```python
from build123d import *

# Parameters (mm, degrees)
SKETCH1_R           = 50.8
BOSS_EXTRUDE1_DEPTH = 15.875
CUT_EXTRUDE2_DEPTH  = 15.24
SKETCH5_R           = 4.191
CUT_EXTRUDE3_DEPTH  = 74.440708058
CUT_EXTRUDE4_DEPTH  = 74.575101937
SKETCH7_R           = 48.26
CUT_EXTRUDE5_DEPTH  = 15.24
SKETCH8_R           = 3.2639
CUT_EXTRUDE6_DEPTH  = 74.575101937


with BuildPart() as part:
    # Sketch1 → Boss-Extrude1 (new body)
    with BuildSketch(Plane(origin=(0, 0, 0), x_dir=(1, 0, 0), z_dir=(0, 1, 0))):
        with Locations(Location((0, 0, 0), (0, 0, 270))):
            Circle(SKETCH1_R)
    extrude(amount=BOSS_EXTRUDE1_DEPTH)

    # Sketch4 → Cut-Extrude2 (cut)
    with BuildSketch(Plane(origin=(0, 15.875, 0), x_dir=(1, 0, 0), z_dir=(0, 1, 0))):
        Polygon((-3.519527241, 6.096), (3.519527241, 6.096), (7.039054482, 0), (3.519527241, -6.096), (-3.519527241, -6.096), (-7.039054482, 0), align=None)
    extrude(amount=-CUT_EXTRUDE2_DEPTH, mode=Mode.SUBTRACT)

    # Sketch5 → Cut-Extrude3 (cut, through all)
    with BuildSketch(Plane(origin=(0, 0.635, 0), x_dir=(1, 0, 0), z_dir=(0, 1, 0))):
        with Locations(Location((0, 0, 0), (0, 0, 270))):
            Circle(SKETCH5_R)
    extrude(amount=-CUT_EXTRUDE3_DEPTH, mode=Mode.SUBTRACT)

    # Sketch6 → Cut-Extrude4 (cut, through all)
    with BuildSketch(Plane(origin=(0, 15.875, 0), x_dir=(1, 0, 0), z_dir=(0, 1, 0))):
        with BuildLine():
            ThreePointArc((-13.470384182, 13.470384182), (-7.290119387, 17.599905094), (0, 19.05))
            Line((0, 19.05), (0, 38.1))
            ThreePointArc((0, 38.1), (-14.580238773, 35.199810189), (-26.940768363, 26.940768363))
            Line((-26.940768363, 26.940768363), (-13.470384182, 13.470384182))
        make_face()
        with BuildLine():
            Line((26.940768363, 26.940768363), (13.470384182, 13.470384182))
            ThreePointArc((13.470384182, 13.470384182), (17.599905094, 7.290119387), (19.05, 0))
            Line((19.05, 0), (38.1, 0))
            ThreePointArc((38.1, 0), (35.199810189, 14.580238773), (26.940768363, 26.940768363))
        make_face()
        with BuildLine():
            Line((26.940768363, -26.940768363), (13.470384182, -13.470384182))
            ThreePointArc((13.470384182, -13.470384182), (7.290119387, -17.599905094), (0, -19.05))
            Line((0, -19.05), (0, -38.1))
            ThreePointArc((0, -38.1), (14.580238773, -35.199810189), (26.940768363, -26.940768363))
        make_face()
        with BuildLine():
            Line((-26.940768363, -26.940768363), (-13.470384182, -13.470384182))
            ThreePointArc((-13.470384182, -13.470384182), (-17.599905094, -7.290119387), (-19.05, 0))
            Line((-19.05, 0), (-38.1, 0))
            ThreePointArc((-38.1, 0), (-35.199810189, -14.580238773), (-26.940768363, -26.940768363))
        make_face()
    extrude(amount=-CUT_EXTRUDE4_DEPTH, mode=Mode.SUBTRACT)

    # Sketch7 → Cut-Extrude5 (cut)
    with BuildSketch(Plane(origin=(0, 15.875, 0), x_dir=(1, 0, 0), z_dir=(0, 1, 0))):
        with Locations(Location((0, 0, 0), (0, 0, 270))):
            Circle(SKETCH7_R)
        with BuildLine():
            Line((-16.313445375, 2.54), (-40.560547334, 2.54))
            ThreePointArc((-40.560547334, 2.54), (-37.546464201, -15.552254691), (-26.884586844, -30.476689292))
            Line((-26.884586844, -30.476689292), (-9.739296625, -13.331399073))
            ThreePointArc((-9.739296625, -13.331399073), (-15.253251082, -6.318103468), (-16.313445375, 2.54))
        make_face(mode=Mode.SUBTRACT)
        with BuildLine():
            Line((16.313445375, -2.54), (40.560547334, -2.54))
            ThreePointArc((40.560547334, -2.54), (37.546464201, 15.552254691), (26.884586844, 30.476689292))
            Line((26.884586844, 30.476689292), (9.739296625, 13.331399073))
            ThreePointArc((9.739296625, 13.331399073), (15.253251082, 6.318103468), (16.313445375, -2.54))
        make_face(mode=Mode.SUBTRACT)
        Polygon((4.985996925, 8.636), (-4.985996925, 8.636), (-9.971993849, 0), (-4.985996925, -8.636), (4.985996925, -8.636), (9.971993849, 0), align=None, mode=Mode.SUBTRACT)
        with BuildLine():
            ThreePointArc((2.54, 40.560547334), (-15.552254691, 37.546464201), (-30.476689292, 26.884586844))
            Line((-30.476689292, 26.884586844), (-13.331399073, 9.739296625))
            ThreePointArc((-13.331399073, 9.739296625), (-6.318103468, 15.253251082), (2.54, 16.313445375))
            Line((2.54, 16.313445375), (2.54, 40.560547334))
        make_face(mode=Mode.SUBTRACT)
        with BuildLine():
            Line((-2.54, -16.313445375), (-2.54, -40.560547334))
            ThreePointArc((-2.54, -40.560547334), (15.552254691, -37.546464201), (30.476689292, -26.884586844))
            Line((30.476689292, -26.884586844), (13.331399073, -9.739296625))
            ThreePointArc((13.331399073, -9.739296625), (6.318103468, -15.253251082), (-2.54, -16.313445375))
        make_face(mode=Mode.SUBTRACT)
    extrude(amount=-CUT_EXTRUDE5_DEPTH, mode=Mode.SUBTRACT)

    # Sketch8 → Cut-Extrude6 (cut, through all)
    with BuildSketch(Plane.XZ):
        with Locations(Location((-35.199810189, -14.580238773, 0), (0, 0, 270))):
            Circle(SKETCH8_R)
        with Locations(Location((35.199810189, 14.580238773, 0), (0, 0, 270))):
            Circle(SKETCH8_R)
        with Locations(Location((14.580238773, -35.199810189, 0), (0, 0, 270))):
            Circle(SKETCH8_R)
        with Locations(Location((-14.580238773, 35.199810189, 0), (0, 0, 270))):
            Circle(SKETCH8_R)
    extrude(amount=-CUT_EXTRUDE6_DEPTH, mode=Mode.SUBTRACT)


solid = part.part
```
Work out the finished part from the listing and answer in its coordinate system (mm). A direction names the side the tool comes from. Round coordinates to 2 decimals unless told otherwise and drop trailing zeros. Loops run counter-clockwise (first coordinate to the right, second up) from the corner with the lowest first, then second, coordinate; pieces in that order, holes last. Notation, with made-up numbers: M 25.25,-35 L 72.25,-35 A23 ccw 72.25,-25 Z; hole C 77.5,42.25 d9. An arc over 180 degrees is marked long. One line per question, with ' | ' between items.
Q1. Find section D-D, the plane z = 36. Give the vertices of the cut face in (x, y) (3 decimals).
Conclusion:
outline: M -35.842,0 L -17.745,0 L -17.745,0.635 L -32.141,0.635 L -32.141,15.875 L -35.842,15.875 Z; M -11.416,0 L 0,0 L 0,15.875 L -2.54,15.875 L -2.54,0.635 L -11.416,0.635 Z; M 12.474,0 L 35.842,0 L 35.842,15.875 L 32.141,15.875 L 32.141,0.635 L 18.858,0.635 L 18.858,15.875 L 12.474,15.875 Z
Q2. The mould has two halves that part along X. Classify faces 4 (the cylindrical face through (-15.204, 8.362, 6.435)), 5 (the flat face through (-19, 15.875, 45)), 6 (the flat face through (20, 8, -20)): +X half, -X half, draft (parallel to the pull), parting line (faces both ways), or undercut.
Conclusion:
face 4: undercut | face 5: draft | face 6: undercut
Q3. Find section B-B, the plane z = -25.5. Give the vertices of the cut face in (x, y) (3 decimals), then the cut area to 3 significant figures.
Conclusion:
outline: M -43.936,0 L -25.5,0 L -25.5,15.875 L -29.092,15.875 L -29.092,0.635 L -40.973,0.635 L -40.973,15.875 L -43.936,15.875 Z; M 0,0 L 25.5,0 L 25.5,15.875 L 21.908,15.875 L 21.908,0.635 L 2.54,0.635 L 2.54,15.875 L 0,15.875 Z; M 28.308,0 L 43.936,0 L 43.936,15.875 L 40.973,15.875 L 40.973,0.635 L 31.644,0.635 L 31.644,15.875 L 28.308,15.875 Z | area: 327 mm2
Q4. A tool of negligible diameter and unlimited length cuts with its end or side. For faces 1 (the flat face through (-5.3, 8.36, -3.01)), 2 (the flat face through (-20, 8, -20)), 3 (the flat face through (-14, 15.875, -36)), from which of +Z, -Z, +X, -X, +Y, -Y can it reach the whole face along a straight path? Write none if from no direction.
Conclusion:
face 1: +Y | face 2: +Y, -Y | face 3: +Z, -Z, +X, -X, +Y
Q5. Find section A-A, the plane y = 3.5. State how many separate pieces and enclosed holes the cut face has, then the cut area to 3 significant figures.
Conclusion:
separate pieces: 6 | enclosed holes: 6 | area: 1,870 mm2
Q6. Each of these flat-tipped pins is pushed along its axis until it touches: pin 1 Ø1 at (x, y) = (39, 11.5) entering from -Z; pin 2 Ø4.5 at (x, y) = (22.5, 5.5) entering from +Z; pin 3 Ø5 at (x, y) = (30, 10) entering from -Z. Where does it stop, or does it pass through?
Conclusion:
pin 1: stops at z = -33.14 | pin 2: stops at z = 46.59 | pin 3: stops at z = -42.71
Q7. Find section C-C, the plane x = 29. Give the vertices of the cut face in (y, z) (3 decimals).
Conclusion:
outline: M 0,-41.709 L 15.875,-41.709 L 15.875,-38.575 L 0.635,-38.575 L 0.635,-28.471 L 15.875,-28.471 L 15.875,-24.711 L 0,-24.711 Z; M 0,0 L 15.875,0 L 15.875,2.54 L 0.635,2.54 L 0.635,25.408 L 15.875,25.408 L 15.875,28.471 L 0.635,28.471 L 0.635,38.575 L 15.875,38.575 L 15.875,41.709 L 0,41.709 Z
Q8. Consider line 1 along X through (y, z) = (4.25, -8); line 2 along X through (y, z) = (0.5, 3); line 3 along X through (y, z) = (9.5, 7.5). Determine where each line is inside the solid, lowest interval first. Write a range as from..to.
Conclusion:
line 1: x = -50.17..-47.59, -5.35..5.35, 14.44..17.29, 37.25..39.84, 47.59..50.17 | line 2: x = -50.71..-37.98, -18.81..-2.93, 2.93..50.71 | line 3: x = -50.24..-47.67, -39.94..-37.35, -17.51..-14.71, -5.64..5.64, 47.67..50.24
